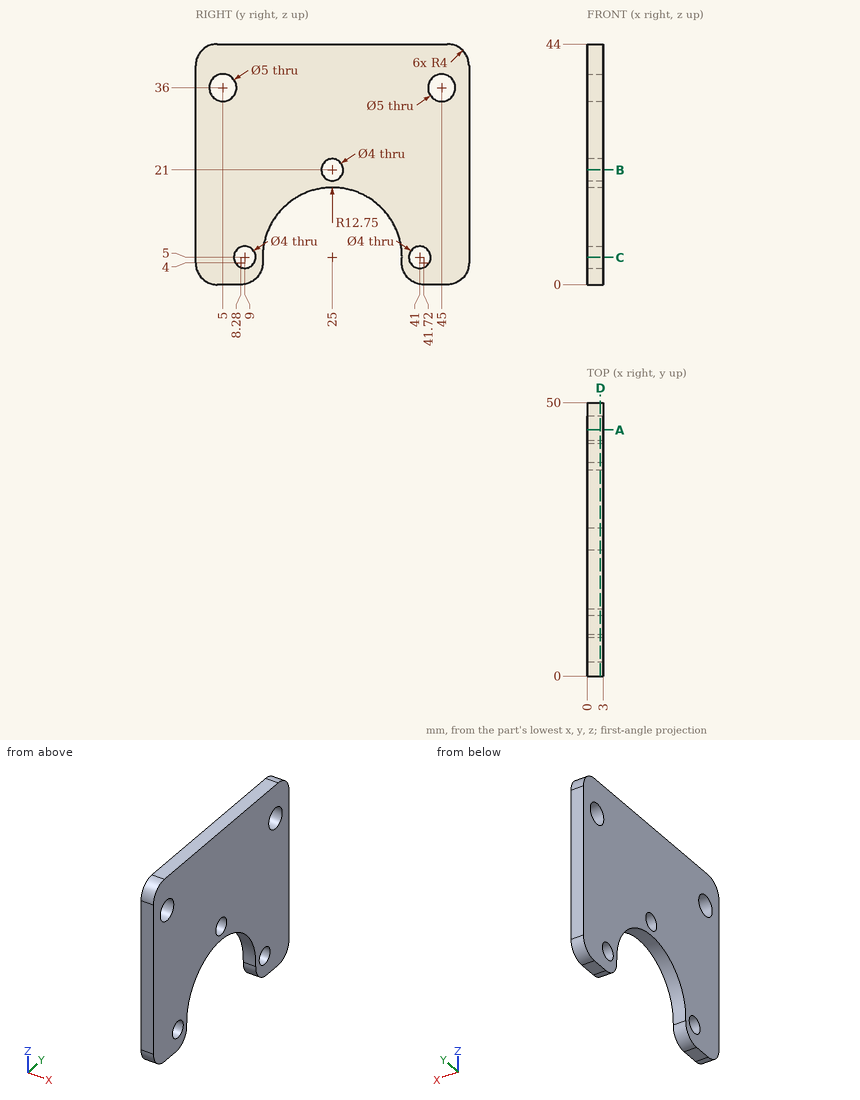
Could you check a few things on this drawing? It's one solid part, dimensions in mm from its lowest x, y, z. Give positions to 0.01 mm unless a question says otherwise; leave off trailing zeros. Loops run counter-clockwise (first coordinate to the right, second up) from the corner with the lowest first, then second, coordinate; pieces in that order, holes last. Notation, with made-up numbers: M 43,58 L 47,58 A35 ccw 47,93 Z; hole C 47.25,-0.5 d1. An arc over 180 degrees is marked long. One line per question, with ' | ' between items. Start each with the question number.
Q1. If I drill on line 1 (Y direction, x = 1.05, z = 5); line 2 (Y direction, x = 1.45, z = 36); line 3 (Y direction, x = 1.8, z = 21), over which ranges is the centre line in solid material (lowest first)? Write a range as from..to.
Q2. If we section it at C-C (z = 5): Please give me the cut outline in (x, y).
Q3. If we section it at D-D (x = 2.45): Please give me the cut outline in (y, z).
Q4. If we section it at A-A (y = 45): Please give me the cut outline in (x, z), plus the area to 3 significant figures.
Q5. For pin 1 Ø3 at (y, z) = (25, 21) entering from -X, with a flat end and sliding along its axis, tell me the tip position at first contact or that it passes through.
Q6. If we section it at B-B (z = 21): Please give me the cut outline in (x, y).
Computed:
1) line 1: y = 0..7, 11..12.25, 37.75..39, 43..50 | line 2: y = 0..2.5, 7.5..42.5, 47.5..50 | line 3: y = 0..23, 27..50
2) outline: M 0,0 L 3,0 L 3,7 L 0,7 Z; M 0,11 L 3,11 L 3,12.25 L 0,12.25 Z; M 0,37.75 L 3,37.75 L 3,39 L 0,39 Z; M 0,43 L 3,43 L 3,50 L 0,50 Z
3) outline: M 0,4 A4 ccw 4,0 L 8.28,0 A4 ccw 12.27,4.24 A12.75 cw long 37.73,4.24 A4 ccw 41.72,0 L 46,0 A4 ccw 50,4 L 50,40 A4 ccw 46,44 L 4,44 A4 ccw 0,40 Z; hole C 5,36 d5; hole C 9,5 d4; hole C 25,21 d4; hole C 41,5 d4; hole C 45,36 d5
4) outline: M 0,0 L 3,0 L 3,33.5 L 0,33.5 Z; M 0,38.5 L 3,38.5 L 3,44 L 0,44 Z | area: 117 mm²
5) pin 1: passes through
6) outline: M 0,0 L 3,0 L 3,23 L 0,23 Z; M 0,27 L 3,27 L 3,50 L 0,50 Z
